from build123d import *

# Parameters (mm, degrees)
BASPROSKE_W              = 15
BASPROSKE_H              = 28.75
TOOTHCUT_DEPTH           = 44.337339558
TEETHCUTS_COUNT          = 21
TEETHCUTS_ANGLE          = 342.857142857
HUBNEAONESKE_R           = 12
HUBNEARONE_DEPTH         = 35.0000508
BORSKE_R                 = 3
BORE_DEPTH               = 15.0000508
CUT_EXTRUDE_1_DEPTH      = 54.627906094
CUT_EXTRUDE_1_DEPTH_BACK = 54.627906094
SKETCH_2_R               = 1.275
CUT_EXTRUDE_2_DEPTH      = 44.312224095
CUT_EXTRUDE_3_DEPTH      = 5


with BuildPart() as part:
    # BasProSke → Base-Revolve (revolve)
    with BuildSketch(Plane(origin=(0, 0, 0), x_dir=(1, 0, 0), z_dir=(0, 1, 0)), mode=Mode.PRIVATE) as base_revolve_sk:
        with Locations((7.5, 14.375)):
            Rectangle(BASPROSKE_W, BASPROSKE_H)
    revolve(base_revolve_sk.sketch.rotate(Axis((-10, 0, 0), (1, 0, 0)), 180), axis=Axis((-10, 0, 0), (1, 0, 0)))

    # TooCutSke → ToothCut (cut, through all)
    with BuildSketch(Plane(origin=(0, 0, 0), x_dir=(0, 0, -1), z_dir=(1, 0, 0))):
        with BuildLine():
            ThreePointArc((1.226021101, 23.091475662), (0, 23.124), (-1.226021101, 23.091475662))
            ThreePointArc((-1.226021101, 23.091475662), (-2.035978165, 25.992768242), (-3.636318743, 28.544716344))
            ThreePointArc((-3.636318743, 28.544716344), (0, 28.7754), (3.636318743, 28.544716344))
            ThreePointArc((3.636318743, 28.544716344), (2.035978165, 25.992768242), (1.226021101, 23.091475662))
        make_face()
    toothcut = extrude(amount=TOOTHCUT_DEPTH, mode=Mode.SUBTRACT)

    # TeethCuts: ToothCut ×21 about axis
    teethcuts_axis = Axis((-10, 0, 0), (1, 0, 0))
    for i in range(1, TEETHCUTS_COUNT):
        add(toothcut.rotate(teethcuts_axis, i * TEETHCUTS_ANGLE / (TEETHCUTS_COUNT - 1)), mode=Mode.SUBTRACT)

    # HubNeaOneSke → HubNearOne (add)
    with BuildSketch(Plane.ZY):
        with Locations(Location((0, 0, 0), (0, 0, 180))):
            Circle(HUBNEAONESKE_R)
    extrude(amount=HUBNEARONE_DEPTH)

    # BorSke → Bore (cut, symmetric)
    with BuildSketch(Plane(origin=(0, 0, 0), x_dir=(0, 0, -1), z_dir=(1, 0, 0))):
        with Locations(Location((0, 0, 0), (0, 0, 180))):
            Circle(BORSKE_R)
    extrude(amount=BORE_DEPTH, both=True, mode=Mode.SUBTRACT)

    # 草圖1 → 除料-伸長1 (cut, two sides: drawn at the far end of the back side and taken through both)
    with BuildSketch(Plane(origin=(0, 0, 0), x_dir=(1, 0, 0), z_dir=(0, 1, 0)).offset(-CUT_EXTRUDE_1_DEPTH_BACK)):
        Polygon((-35.0000508, -11.862952099), (-35.0000508, -15.448809423), (0, -15.448809423), (0, -11.862952099), (0, 12), (-35.0000508, 12), align=None)
    extrude(amount=CUT_EXTRUDE_1_DEPTH + CUT_EXTRUDE_1_DEPTH_BACK, mode=Mode.SUBTRACT)

    # 草圖2 → 除料-伸長2 (cut, through all)
    with BuildSketch(Plane.ZY):
        with Locations((0, 8)):
            Circle(SKETCH_2_R)
        with Locations((8, 0)):
            Circle(SKETCH_2_R)
        with Locations((0, -8)):
            Circle(SKETCH_2_R)
        with Locations((-8, 0)):
            Circle(SKETCH_2_R)
    extrude(amount=-CUT_EXTRUDE_2_DEPTH, mode=Mode.SUBTRACT)

    # 草圖3 → 除料-伸長3 (cut)
    with BuildSketch(Plane.ZY):
        with BuildLine():
            ThreePointArc((15.633632839, -24.127826762), (16.195451669, -23.754364762), (16.748353108, -23.367823351))
            ThreePointArc((16.748353108, -23.367823351), (16.182150595, -20.424548747), (14.807455158, -17.761155586))
            ThreePointArc((14.807455158, -17.761155586), (15.728314388, -16.951091484), (16.604929283, -16.093343329))
            ThreePointArc((16.604929283, -16.093343329), (19.158143938, -17.66323046), (22.050876182, -18.447800942))
            ThreePointArc((22.050876182, -18.447800942), (22.477655121, -17.925331803), (22.892057619, -17.392992783))
            ThreePointArc((22.892057619, -17.392992783), (21.483464476, -14.747370732), (19.384793984, -12.60750325))
            ThreePointArc((19.384793984, -12.60750325), (20.025971437, -11.562), (20.610815085, -10.483972412))
            ThreePointArc((20.610815085, -10.483972412), (23.513329931, -11.231540632), (26.508802408, -11.128607052))
            ThreePointArc((26.508802408, -11.128607052), (26.762620274, -10.503554451), (27.001702351, -9.872718478))
            ThreePointArc((27.001702351, -9.872718478), (24.87587826, -7.75982411), (22.239708796, -6.333618923))
            ThreePointArc((22.239708796, -6.333618923), (22.544233041, -5.145574077), (22.785339517, -3.943054539))
            ThreePointArc((22.785339517, -3.943054539), (25.779253374, -3.80187913), (28.611305207, -2.820587588))
            ThreePointArc((28.611305207, -2.820587588), (28.669609169, -2.148490191), (28.712127333, -1.475209811))
            ThreePointArc((28.712127333, -1.475209811), (26.057961094, -0.082783062), (23.118527885, 0.50303524))
            ThreePointArc((23.118527885, 0.50303524), (23.059340606, 1.728058684), (22.935286541, 2.948221034))
            ThreePointArc((22.935286541, 2.948221034), (25.754577023, 3.965596017), (28.17156798, 5.738053461))
            ThreePointArc((28.17156798, 5.738053461), (28.029177475, 6.397476851), (27.871353801, 7.053377721))
            ThreePointArc((27.871353801, 7.053377721), (24.924679732, 7.601613624), (21.943164316, 7.294992515))
            ThreePointArc((21.943164316, 7.294992515), (21.525524564, 8.448145847), (21.047332707, 9.57753423))
            ThreePointArc((21.047332707, 9.57753423), (23.441493482, 11.380710555), (25.22866331, 13.786843279))
            ThreePointArc((25.22866331, 13.786843279), (24.898230359, 14.375), (24.554088173, 14.95524169))
            ThreePointArc((24.554088173, 14.95524169), (21.576731195, 14.610573581), (18.818054303, 13.438757691))
            ThreePointArc((18.818054303, 13.438757691), (18.079071201, 14.417578178), (17.289230996, 15.35584148))
            ThreePointArc((17.289230996, 15.35584148), (19.045530374, 17.784599017), (20.04408119, 20.610611569))
            ThreePointArc((20.04408119, 20.610611569), (19.554966211, 21.075241315), (19.055084056, 21.528266805))
            ThreePointArc((19.055084056, 21.528266805), (16.311595404, 20.321319958), (14.020877582, 18.388430271))
            ThreePointArc((14.020877582, 18.388430271), (13.026213023, 19.105945417), (11.994905239, 19.769714826))
            ThreePointArc((11.994905239, 19.769714826), (12.957288312, 22.608247809), (13.078494494, 25.603036573))
            ThreePointArc((13.078494494, 25.603036573), (12.4741575, 25.902854952), (11.862952099, 26.188410939))
            ThreePointArc((11.862952099, 26.188410939), (9.597102778, 24.226427877), (7.977884359, 21.704210125))
            ThreePointArc((7.977884359, 21.704210125), (6.815918653, 22.096665561), (5.634779513, 22.426962252))
            ThreePointArc((5.634779513, 22.426962252), (5.717734322, 25.42305457), (4.950826169, 28.320519421))
            ThreePointArc((4.950826169, 28.320519421), (4.284965153, 28.428886254), (3.616744788, 28.521599835))
            ThreePointArc((3.616744788, 28.521599835), (2.029865455, 25.978911364), (1.226021101, 23.091475662))
            ThreePointArc((1.226021101, 23.091475662), (0, 23.124), (-1.226021101, 23.091475662))
            ThreePointArc((-1.226021101, 23.091475662), (-2.029865455, 25.978911364), (-3.616744788, 28.521599835))
            ThreePointArc((-3.616744788, 28.521599835), (-4.284965153, 28.428886254), (-4.950826169, 28.320519421))
            ThreePointArc((-4.950826169, 28.320519421), (-5.717734322, 25.42305457), (-5.634779513, 22.426962252))
            ThreePointArc((-5.634779513, 22.426962252), (-6.815918653, 22.096665561), (-7.977884359, 21.704210125))
            ThreePointArc((-7.977884359, 21.704210125), (-9.597102778, 24.226427877), (-11.862952099, 26.188410939))
            ThreePointArc((-11.862952099, 26.188410939), (-12.4741575, 25.902854952), (-13.078494494, 25.603036573))
            ThreePointArc((-13.078494494, 25.603036573), (-12.957288312, 22.608247809), (-11.994905239, 19.769714826))
            ThreePointArc((-11.994905239, 19.769714826), (-13.026213023, 19.105945417), (-14.020877582, 18.388430271))
            ThreePointArc((-14.020877582, 18.388430271), (-16.311595404, 20.321319958), (-19.055084056, 21.528266805))
            ThreePointArc((-19.055084056, 21.528266805), (-19.554966211, 21.075241315), (-20.04408119, 20.610611569))
            ThreePointArc((-20.04408119, 20.610611569), (-19.045530374, 17.784599017), (-17.289230996, 15.35584148))
            ThreePointArc((-17.289230996, 15.35584148), (-18.079071201, 14.417578178), (-18.818054303, 13.438757691))
            ThreePointArc((-18.818054303, 13.438757691), (-21.576731195, 14.610573581), (-24.554088173, 14.95524169))
            ThreePointArc((-24.554088173, 14.95524169), (-24.898230359, 14.375), (-25.22866331, 13.786843279))
            ThreePointArc((-25.22866331, 13.786843279), (-23.441493482, 11.380710555), (-21.047332707, 9.57753423))
            ThreePointArc((-21.047332707, 9.57753423), (-21.525524564, 8.448145847), (-21.943164316, 7.294992515))
            ThreePointArc((-21.943164316, 7.294992515), (-24.924679732, 7.601613624), (-27.871353801, 7.053377721))
            ThreePointArc((-27.871353801, 7.053377721), (-28.029177475, 6.397476851), (-28.17156798, 5.738053461))
            ThreePointArc((-28.17156798, 5.738053461), (-25.754577023, 3.965596017), (-22.935286541, 2.948221034))
            ThreePointArc((-22.935286541, 2.948221034), (-23.059340606, 1.728058684), (-23.118527885, 0.50303524))
            ThreePointArc((-23.118527885, 0.50303524), (-26.057961094, -0.082783062), (-28.712127333, -1.475209811))
            ThreePointArc((-28.712127333, -1.475209811), (-28.669609169, -2.148490191), (-28.611305207, -2.820587588))
            ThreePointArc((-28.611305207, -2.820587588), (-25.779253374, -3.80187913), (-22.785339517, -3.943054539))
            ThreePointArc((-22.785339517, -3.943054539), (-22.544233041, -5.145574077), (-22.239708796, -6.333618923))
            ThreePointArc((-22.239708796, -6.333618923), (-24.87587826, -7.75982411), (-27.001702351, -9.872718478))
            ThreePointArc((-27.001702351, -9.872718478), (-26.762620274, -10.503554451), (-26.508802408, -11.128607052))
            ThreePointArc((-26.508802408, -11.128607052), (-23.513329931, -11.231540632), (-20.610815085, -10.483972412))
            ThreePointArc((-20.610815085, -10.483972412), (-20.025971437, -11.562), (-19.384793984, -12.60750325))
            ThreePointArc((-19.384793984, -12.60750325), (-21.483464476, -14.747370732), (-22.892057619, -17.392992783))
            ThreePointArc((-22.892057619, -17.392992783), (-22.477655121, -17.925331803), (-22.050876182, -18.447800942))
            ThreePointArc((-22.050876182, -18.447800942), (-19.158143938, -17.66323046), (-16.604929283, -16.093343329))
            ThreePointArc((-16.604929283, -16.093343329), (-15.728314388, -16.951091484), (-14.807455158, -17.761155586))
            ThreePointArc((-14.807455158, -17.761155586), (-16.182150595, -20.424548747), (-16.748353108, -23.367823351))
            ThreePointArc((-16.748353108, -23.367823351), (-16.195451669, -23.754364762), (-15.633632839, -24.127826762))
            ThreePointArc((-15.633632839, -24.127826762), (-13.100672782, -22.525464747), (-11.123622645, -20.272750066))
            ThreePointArc((-11.123622645, -20.272750066), (-10.033127583, -20.834004101), (-8.914408959, -21.336651305))
            ThreePointArc((-8.914408959, -21.336651305), (-9.44298162, -24.286915974), (-9.116483925, -27.266320266))
            ThreePointArc((-9.116483925, -27.266320266), (-8.474211264, -27.472718166), (-7.827272612, -27.663989291))
            ThreePointArc((-7.827272612, -27.663989291), (-5.879149357, -25.386212641), (-4.65393332, -22.650833995))
            ThreePointArc((-4.65393332, -22.650833995), (-3.446453363, -22.865724026), (-2.229278404, -23.016291921))
            ThreePointArc((-2.229278404, -23.016291921), (-1.864762288, -25.991284136), (-0.674575137, -28.742084969))
            ThreePointArc((-0.674575137, -28.742084969), (0, -28.75), (0.674575137, -28.742084969))
            ThreePointArc((0.674575137, -28.742084969), (1.864762288, -25.991284136), (2.229278404, -23.016291921))
            ThreePointArc((2.229278404, -23.016291921), (3.446453363, -22.865724026), (4.65393332, -22.650833995))
            ThreePointArc((4.65393332, -22.650833995), (5.879149357, -25.386212641), (7.827272612, -27.663989291))
            ThreePointArc((7.827272612, -27.663989291), (8.474211264, -27.472718166), (9.116483925, -27.266320266))
            ThreePointArc((9.116483925, -27.266320266), (9.44298162, -24.286915974), (8.914408959, -21.336651305))
            ThreePointArc((8.914408959, -21.336651305), (10.033127583, -20.834004101), (11.123622645, -20.272750066))
            ThreePointArc((11.123622645, -20.272750066), (13.100672782, -22.525464747), (15.633632839, -24.127826762))
        make_face()
    extrude(amount=-CUT_EXTRUDE_3_DEPTH, mode=Mode.SUBTRACT)


solid = part.part
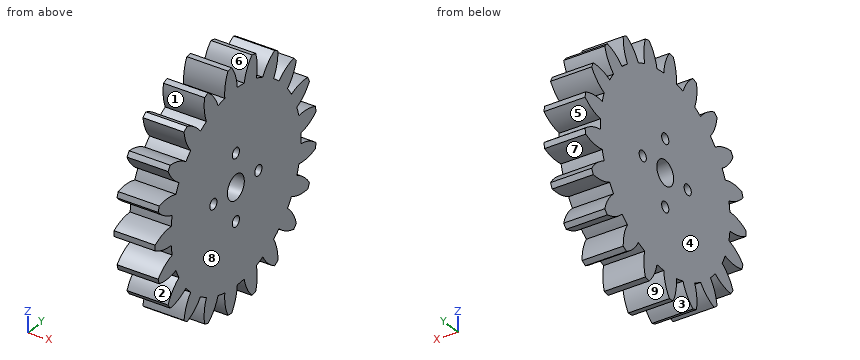
Design review of the part built by this model. Coordinates are the model's own, in mm. Face numbers are marked on the shaded views. A direction names the side the tool comes from. Give positions to 0.01 mm unless a question says otherwise; leave off trailing zeros. Loops run counter-clockwise (first coordinate to the right, second up) from the corner with the lowest first, then second, coordinate; pieces in that order, holes last. Notation, with made-up numbers: (-2, -4.5) - (43, -4.5) arc R24 ccw to (43, 30.5) - close; hole circle Ø4 at (57, -39). An arc over 180 degrees is marked (long way). Use CSV: the item, a comma, the result in double quotes. Start each with the question number.
1. Add section A-A (z = 0). State the section outline as (x, y) points (3 decimals).
2. Draft analysis for pull direction Z (two halves, no side actions). For the marked faces 6, 7, 8 and 9, state which applies: released by +Z, released by -Z, zero draft, split by the parting line, or undercut.
3. Machinability: for the marked faces 1, 2, 3, 4 and 5, which of the approach directions +Z, -Z, +X, -X, +Y, -Y give a long, thin tool a straight path to every point of the face, cutting with its end or side? Answer none if there is none.
4. Add section C-C (y = -14). State the section outline as (x, z) points.
5. Insertion check: P1, Ø6, axis at x = 13.5, y = -17, coming from the +Z side; P2, Ø6, axis at x = 12, y = 16.5, coming from the +Z side. Each pin has a flat end and moves straight along its axis. Give the tip position at first contact, or say it passes through.
6. Wall thickness on L1, parallel to Y at x = 12.25, z = 0 (3 decimals); L2, parallel to Z at x = 8, y = 25; L3, parallel to Y at x = 13.5, z = -15: over which ranges is each line inside the solid? List them lowest first.
7. Add section B-B (x = 10.75). Count the separate pieces of the cut face and the enclosed holes in it, plus the area to 3 significant figures.
Results found:
1,outline,"(5, -28.75) - (15, -28.75) - (15, -9.275) - (5, -9.275) - close; (5, -6.725) - (15, -6.725) - (15, -3) - (5, -3) - close; (5, 3) - (15, 3) - (15, 6.725) - (5, 6.725) - close; (5, 9.275) - (15, 9.275) - (15, 23.124) - (5, 23.124) - close"
2,face 6,"released by +Z"
2,face 7,"undercut"
2,face 8,"zero draft"
2,face 9,"released by -Z"
3,face 1,"+X, -X"
3,face 2,"+X, -X, -Y"
3,face 3,"-Z, +X, -X"
3,face 4,"+Z, -Z, -X, +Y, -Y"
3,face 5,"+X, -X, +Y"
4,outline,"(5, -20.88) - (15, -20.88) - (15, 20.88) - (5, 20.88) - close"
5,P1,"stops at z = 22.89"
5,P2,"stops at z = 25.23"
6,L1,"y = -28.75 to -9.275, -6.725 to -3, 3 to 6.725, 9.275 to 23.124"
6,L2,"z = -13.12 to -10.34, -5.76 to -1.66, 1.66 to 5.76, 10.34 to 13.12"
6,L3,"y = -23.82 to -18.04, -17.6 to 19.35"
7,separate pieces,"1"
7,enclosed holes,"5"
7,area,"2,050 mm²"
